from build123d import *

# Parameters (mm, degrees)
F0_W     = 50
F0_H     = 3
F1_DEPTH = 7.5
F2_W     = 35
F2_H     = 10
F3_DEPTH = 1.5
F5_D     = 2


with BuildPart() as f1:
    # F0 (on Front) → F1 (new body, symmetric)
    with BuildSketch(Plane.XZ):
        Rectangle(F0_W, F0_H)
    extrude(amount=F1_DEPTH, both=True)

    # F2 (on Top) → F3 (cut, symmetric)
    with BuildSketch(Plane.XY):
        with Locations((5, 0)):
            Rectangle(F2_W, F2_H)
    extrude(amount=F3_DEPTH, both=True, mode=Mode.SUBTRACT)

    # F5 (through all)
    with Locations(Plane.XZ.offset(7.5)):
        with Locations((5, 0)):
            Hole(F5_D / 2)


solid = f1.part
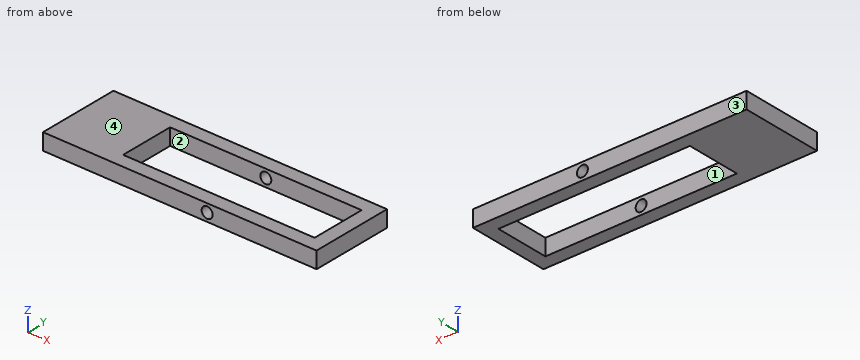
The listing builds one solid part. Answer for the finished solid, in the listing's coordinates (mm). Face numbers are marked on the shaded views. Coordinates: 2 decimals unless noted, no trailing zeros. Order: outer loops, then holes, each group sorted by start corner. A loop starts at its lowest first (then second) coordinate and runs counter-clockwise, first axis right, second up.
Q1. Given P1, Ø1.6, axis at x = 5, z = 0, coming from the +Y side, flat-ended and moving along its own axis, determine where the tip first touches the part or whether it passes through.
Q2. For a pull along Y with two mould halves and no side action, classify the marked faces 1, 2, 3 and 4 as pulls with the +Y half, pulls with the -Y half, needs draft (parallel to the pull), parting line crosses it, or undercut.
Q3. Consider line 1 (Z direction, x = 5, y = -5.7); line 2 (Y direction, x = 16, z = 1.1); line 3 (X direction, y = 0.25, z = -0.1). Determine where each line is inside the solid, lowest interval first.
Q4. A cutting plane is placed at C-C, the plane x = 2.5. Write down the section's boundary in (y, z).
Q5. A cutting plane is placed at A-A, the plane y = -4.5. Write down the section's boundary in (x, z).
Q6. A cutting plane is placed at B-B, the plane z = 0. Write down the section's boundary in (x, y).
Answers follow:
1. P1: passes through
2. face 1: undercut
2. face 2: undercut
2. face 3: pulls with the +Y half
2. face 4: needs draft
3. line 1: z = -1.5 to -1, 1 to 1.5
3. line 2: y = -7.5 to -5, 5 to 7.5
3. line 3: x = -25 to -12.5, 22.5 to 25
4. outline: (-7.5, -1.5) - (-5, -1.5) - (-5, 1.5) - (-7.5, 1.5) - close; (5, -1.5) - (7.5, -1.5) - (7.5, 1.5) - (5, 1.5) - close
5. outline: (-25, -1.5) - (-12.5, -1.5) - (-12.5, 1.5) - (-25, 1.5) - close; (22.5, -1.5) - (25, -1.5) - (25, 1.5) - (22.5, 1.5) - close
6. outline: (-25, -7.5) - (4, -7.5) - (4, -5) - (-12.5, -5) - (-12.5, 5) - (4, 5) - (4, 7.5) - (-25, 7.5) - close; (6, -7.5) - (25, -7.5) - (25, 7.5) - (6, 7.5) - (6, 5) - (22.5, 5) - (22.5, -5) - (6, -5) - close
